Part model, mm, in its own coordinate system. A direction names the side the tool comes from. Round coordinates to 2 decimals unless told otherwise and drop trailing zeros. Loops run counter-clockwise (first coordinate to the right, second up) from the corner with the lowest first, then second, coordinate; pieces in that order, holes last.
Autodesk Fusion 360 part; units mm, degrees
sketch "Sketch1" plane through (0, 0, 0) normal (0, -1, 0) x (1, 0, 0) in component "DDD Wall Control Center Piece Parametric Template"
  line L0 (11.6, -25.3) -> (-11.6, -25.3)
  line L1 (-11.6, -25.3) -> (-11.6, 25.3)
  line L2 (-11.6, 25.3) -> (11.6, 25.3)
  line L3 (11.6, 25.3) -> (11.6, -25.3)
  line L4 (11.6, -25.3) -> (-11.6, 25.3) construction
  line L5 (-11.6, -25.3) -> (11.6, 25.3) construction
  dimension "d1" = 23.2
  dimension "d2" = 50.6
extrude "Extrude1" add sketch "Sketch1" against normal blind 8.7 in component "DDD Wall Control Center Piece Parametric Template"
sketch "Sketch3" plane through (0, 0, 0) normal (1, 0, 0) x (0, 0, 1) in component "DDD Wall Control Center Piece Parametric Template"
  line L0 (-17.7, -2.35) -> (-7.7, -2.35)
  line L1 (-7.7, -2.35) -> (-7.7, -6.35)
  line L2 (-7.7, -6.35) -> (-17.7, -6.35)
  line L3 (-17.7, -6.35) -> (-17.7, -2.35)
  line L4 (-17.7, -2.35) -> (-7.7, -6.35) construction
  line L5 (-7.7, -2.35) -> (-17.7, -6.35) construction
  line L6 (1.75, 0) -> (22.5, 0)
  line L7 (25.3, 0) -> (-25.3, 0)
  point P0 (-12.7, -4.35)
  dimension "d165" = 10
  dimension "d166" = 4
  dimension "d189" = 17.7
  dimension "d205" = 2.35
extrude "Extrude3" cut sketch "Sketch3" against normal blind 4 from surface at 11.6 in component "DDD Wall Control Center Piece Parametric Template"
mirror "Mirror2" about plane through (0, 0, 0) normal (1, 0, 0) of "Extrude3" in component "DDD Wall Control Center Piece Parametric Template"
pattern_linear "R-Pattern4" count 2 spacing 25.4 along (0, 0, 1) of "Extrude3" in component "DDD Wall Control Center Piece Parametric Template"
mirror "Mirror1" about plane through (0, 0, 0) normal (1, 0, 0) of "R-Pattern4" in component "DDD Wall Control Center Piece Parametric Template"
component "DDD Wall Control Center Piece Parametric Template" placed x (1, 0, 0) y (0, 1, 0) z (0, 0, 1) at (0, 0, 0)
equation "d1 = HorizontalWidth"
equation "d2 = VerticalHeight"
equation "d42 = -PinHoleWidth / 2"
equation "d165 = PinHoleLength"
equation "d166 = PinHoleHeight"
equation "SidepieceDepth = 8.7 mm"
equation "HorizontalWidthBetweenSlots = SlotSpacing - SlotWidth"
equation "PinHoleLength = 10 mm"
equation "PinHoleWidth = 8 mm"
equation "PinHoleHeight = 4 mm"
equation "SlotSpacing = 25.4 mm"
equation "PinToEdgeLength = 7.6 mm"
equation "HorizontalWidth = ( HorizontalUnits - 1 ) * SlotSpacing + HorizontalWidthBetweenSlots"
equation "VerticalHeight = ( VerticalUnits - 1 ) * SlotSpacing + PinHoleLength + 2 * PinToEdgeLength"
equation "d189 = ( VerticalHeight / 2 ) - PinToEdgeLength"
equation "Depth = max(DepthOverride; PinHoleHeight + PinDepthOffset * 2)"
equation "SlotWidth = 2.2 mm"
equation "DepthOverride = 0 mm"
equation "PinDepthOffset = ( SidepieceDepth - PinHoleHeight ) / 2"
equation "d205 = PinDepthOffset"
1) Slice it at A-A, the plane x = 9.5. Give the cut face in (y, z).
Values:
outline: (0, -25.3) - (8.7, -25.3) - (8.7, 25.3) - (0, 25.3) - close; hole (2.35, -17.7) - (6.35, -17.7) - (6.35, -7.7) - (2.35, -7.7) - close; hole (2.35, 7.7) - (6.35, 7.7) - (6.35, 17.7) - (2.35, 17.7) - close
2) Mould opens along Y. For faces 1 (the face through (0, 8.7, 0)), 2 (the face through (-10, 2.35, 13)), 3 (the face through (0, 4, 25.3)) say: released by +Y, released by -Y, zero draft, split by the parting line, or undercut.
Values:
face 1: released by +Y
face 2: undercut
face 3: zero draft
3) Slice it at C-C, the plane z = -12. Give the cut face in (x, y), then the cut area to 3 significant figures.
Values:
outline: (-11.6, 0) - (11.6, 0) - (11.6, 2.35) - (7.6, 2.35) - (7.6, 6.35) - (11.6, 6.35) - (11.6, 8.7) - (-11.6, 8.7) - (-11.6, 6.35) - (-7.6, 6.35) - (-7.6, 2.35) - (-11.6, 2.35) - close
area: 170 mm2
4) Slice it at B-B, the plane y = 3.25. Give the cut face in (x, z).
Values:
outline: (-11.6, -25.3) - (11.6, -25.3) - (11.6, -17.7) - (7.6, -17.7) - (7.6, -7.7) - (11.6, -7.7) - (11.6, 7.7) - (7.6, 7.7) - (7.6, 17.7) - (11.6, 17.7) - (11.6, 25.3) - (-11.6, 25.3) - (-11.6, 17.7) - (-7.6, 17.7) - (-7.6, 7.7) - (-11.6, 7.7) - (-11.6, -7.7) - (-7.6, -7.7) - (-7.6, -17.7) - (-11.6, -17.7) - close
5) Tool access for faces 4 (the face through (-10, 2.35, -13)), 5 (the face through (-11.6, 4, 0)), 6 (the face through (10, 4, -7.7)): list every direction of +Z, -Z, +X, -X, +Y, -Y with a clear straight run to the whole face (end or side of a thin tool).
Values:
face 4: -X
face 5: +Z, -Z, -X, +Y, -Y
face 6: +X
6) Wall check: line 1 along Z through (x, y) = (-8.5, 4.25); line 2 along Y through (x, z) = (7.75, 17.5); line 3 along X through (y, z) = (4.25, 16.5). Give the ranges that are in metal, low to high.
Values:
line 1: z = -25.3 to -17.7, -7.7 to 7.7, 17.7 to 25.3
line 2: y = 0 to 2.35, 6.35 to 8.7
line 3: x = -7.6 to 7.6
